Autodesk Inventor part; units mm, degrees
ref_plane "YZ Plane" through (0, 0, 0) normal (1, 0, 0) x (0, 1, 0)
ref_plane "XZ Plane" through (0, 0, 0) normal (0, 1, 0) x (-1, 0, 0)
ref_plane "XY Plane" through (0, 0, 0) normal (0, 0, 1) x (1, 0, 0)
sketch "Sketch1" plane through (0, 0, 0) normal (0, 0, 1) x (1, 0, 0)
  line L0 (-49.5, 60.5) -> (49.5, 60.5)
  line L1 (49.5, 60.5) -> (49.5, -60.5)
  line L2 (49.5, -60.5) -> (-49.5, -60.5)
  line L3 (-49.5, -60.5) -> (-49.5, 60.5)
  line L4 (-49.5, 60.5) -> (49.5, -60.5) construction
  line L5 (49.5, 60.5) -> (-49.5, -60.5) construction
  point P0 (0, 0)
  dimension "d0" = 99
  dimension "d1" = 121
extrude "Extrusion1" add sketch "Sketch1" along normal blind 2
sketch "Sketch2" plane through (0, 0, 2) normal (0, 0, 1) x (1, 0, 0)
  line L0 (-47.3, 58.3) -> (47.3, 58.3)
  line L1 (47.3, 58.3) -> (47.3, -58.3)
  line L2 (47.3, -58.3) -> (-47.3, -58.3)
  line L3 (-47.3, -58.3) -> (-47.3, 58.3)
  line L4 (-47.3, 58.3) -> (47.3, -58.3) construction
  line L5 (47.3, 58.3) -> (-47.3, -58.3) construction
  point P0 (0, 0)
  dimension "d4" = 116.6
  dimension "d5" = 94.6
extrude "Extrusion2" add sketch "Sketch2" along normal blind 3
fillet "Fillet1" radius 2 4 edges at (49.5, 60.5, 1) (-49.5, 60.5, 1) (49.5, -60.5, 1) (-49.5, -60.5, 1)
sketch "Sketch5" plane through (0, 0, 5) normal (0, 0, 1) x (1, 0, 0)
  line L0 (44.3, -55.3) -> (-44.3, -55.3)
  line L1 (-44.3, -55.3) -> (-44.3, 55.3)
  line L2 (-44.3, 55.3) -> (44.3, 55.3)
  line L3 (44.3, 55.3) -> (44.3, -55.3)
  line L4 (44.3, -55.3) -> (-44.3, 55.3) construction
  line L5 (-44.3, -55.3) -> (44.3, 55.3) construction
  line L6 (47.3, 58.3) -> (-47.3, 58.3)
  line L7 (47.3, -58.3) -> (47.3, 58.3)
  line L8 (-78.6, 90.6) -> (-10, 90.6)
  line L9 (-10, 90.6) -> (-10, 20)
  line L10 (-10, 20) -> (-78.6, 20)
  line L11 (-78.6, 20) -> (-78.6, 90.6)
  line L12 (-78.6, 90.6) -> (-10, 20) construction
  line L13 (-10, 90.6) -> (-78.6, 20) construction
  line L14 (78.6, 90.6) -> (10, 90.6)
  line L15 (10, 90.6) -> (10, 20)
  line L16 (10, 20) -> (78.6, 20)
  line L17 (78.6, 20) -> (78.6, 90.6)
  line L18 (78.6, 90.6) -> (10, 20) construction
  line L19 (10, 90.6) -> (78.6, 20) construction
  line L20 (10, -20) -> (78.6, -20)
  line L21 (78.6, -20) -> (78.6, -90.6)
  line L22 (78.6, -90.6) -> (10, -90.6)
  line L23 (10, -90.6) -> (10, -20)
  line L24 (10, -20) -> (78.6, -90.6) construction
  line L25 (78.6, -20) -> (10, -90.6) construction
  line L26 (-78.6, -90.6) -> (-10, -90.6)
  line L27 (-10, -90.6) -> (-10, -20)
  line L28 (-10, -20) -> (-78.6, -20)
  line L29 (-78.6, -20) -> (-78.6, -90.6)
  line L30 (-78.6, -90.6) -> (-10, -20) construction
  line L31 (-10, -90.6) -> (-78.6, -20) construction
  point P0 (0, 0)
  point P1 (-10, -55.3)
  point P2 (-44.3, -20)
  point P3 (44.3, -20)
  point P4 (10, -55.3)
  point P5 (-44.3, 20)
  point P6 (-10, 55.3)
  point P7 (10, 55.3)
  point P8 (44.3, 20)
  dimension "d23" = 3
  dimension "d24" = 3
  dimension "d27" = 20
  dimension "d28" = 40
extrude "Extrusion5" cut sketch "Sketch5" against normal up to surface (3 mm away) contours L3 L20 L21 L22 L23 L0 | L0 L23 L20 L3 | L0 L27 L28 L1 L10 L9 L2 L15 L16 L3 L20 L23 | L27 L26 L29 L28 L1 L0 | L0 L1 L28 L27 | L16 L15 L2 L3 | L3 L2 L15 L6 L7 L16 | L7 L6 L15 L14 L17 L16 | L10 L11 L8 L9 L2 L1 | L1 L2 L9 L10
equation "\"BendRadius\" = Thickness"
equation "\"BendReliefWidth\" = Thickness"
equation "\"BendReliefDepth\" = 0.5 * Thickness"
equation "\"CornerReliefSize\" = 4 * Thickness"
equation "\"MinimumRemnant\" = 2 * Thickness"
equation "\"TransitionRadius\" = BendRadius"
equation "\"JacobiRadiusSize\" = BendRadius"
equation "\"GapSize\" = Thickness"
properties part number "_3DPrint"
Geometry: final body of the model. Coordinates: model frame, mm. A direction names the side the tool comes from. Give positions to 0.01 mm unless a question says otherwise; leave off trailing zeros. Loops run counter-clockwise (first coordinate to the right, second up) from the corner with the lowest first, then second, coordinate; pieces in that order, holes last. Notation, with made-up numbers: (47.25, 56) - (61.25, 56) arc R13 ccw to (61.25, 81) - close; hole circle Ø11 at (44, 24). An arc over 180 degrees is marked (long way). One line per question, with ' | ' between items. Start each with the question number.
(1) Ray query, line 1 (X direction, y = 4.5, z = 3.6); line 2 (Y direction, x = 1, z = 2.6); line 3 (Z direction, x = 21.5, y = -35.5). Return the intervals inside material, ascending. Write a range as from..to.
(2) Reachability of faces 5 (the flat face through (47.3, 0, 3)), 6 (the flat face through (-44.3, 0, 4)), 7 (the flat face through (0, -58.3, 3)), 8 (the flat face through (-47.3, 0, 3)) from +Z, -Z, +X, -X, +Y, -Y: full face, straight path, thin tool, end or side. Return the list, or none.
(3) Section query C-C on y = -4.5. Return loops of the section in (x, z), then the cut area to 3 significant figures.
(4) Section query D-D on y = -37.5. Return loops of the section in (x, z).
(5) Section query B-B on x = 7. Return loops of the section in (y, z).
(6) Pull-direction query (Y, two-part tool) for faces 1 (the flat face through (46, -20, 4)), 2 (the flat face through (0, 58.3, 3)), 3 (the flat face through (10, 57, 4)), 4 (the flat face through (0, 55.3, 4)); classes: released by +Y, released by -Y, zero draft, split by the parting line, or undercut.
(7) Contact query for flat-ended pins moving along their axis: pin 1 (1.5 mm diameter, centred on x = 46.5, z = 3, fed in from -Y); pin 2 (0.9 mm diameter, centred on x = 1, z = 3, fed in from +Y); pin 3 (1 mm diameter, centred on x = -39.5, z = 4, fed in from +Y); pin 4 (2.5 mm diameter, centred on y = -2, z = 3, fed in from +X). Output: stop coordinate, or through.
(8) Section query A-A on z = 3. Return loops of the section in (x, y), then the cut area to 3 significant figures.
The answers:
1) line 1: -47.3..-44.3, 44.3..47.3 | line 2: -58.3..-55.3, 55.3..58.3 | line 3: 0..2
2) face 5: +Z, +X, +Y, -Y | face 6: +Z, +Y, -Y | face 7: +Z, +X, -X, -Y | face 8: +Z, -X, +Y, -Y
3) outline: (-49.5, 0) - (49.5, 0) - (49.5, 2) - (47.3, 2) - (47.3, 5) - (44.3, 5) - (44.3, 2) - (-44.3, 2) - (-44.3, 5) - (-47.3, 5) - (-47.3, 2) - (-49.5, 2) - close | area: 216 mm2
4) outline: (-49.5, 0) - (49.5, 0) - (49.5, 2) - (-49.5, 2) - close
5) outline: (-60.5, 0) - (60.5, 0) - (60.5, 2) - (58.3, 2) - (58.3, 5) - (55.3, 5) - (55.3, 2) - (-55.3, 2) - (-55.3, 5) - (-58.3, 5) - (-58.3, 2) - (-60.5, 2) - close
6) face 1: released by -Y | face 2: released by +Y | face 3: zero draft | face 4: undercut
7) pin 1: y = -20 | pin 2: y = 58.3 | pin 3: through | pin 4: x = 49.5
8) outline: (-47.3, -20) - (-44.3, -20) - (-44.3, 20) - (-47.3, 20) - close; (-10, -58.3) - (10, -58.3) - (10, -55.3) - (-10, -55.3) - close; (-10, 55.3) - (10, 55.3) - (10, 58.3) - (-10, 58.3) - close; (44.3, -20) - (47.3, -20) - (47.3, 20) - (44.3, 20) - close | area: 360 mm2
